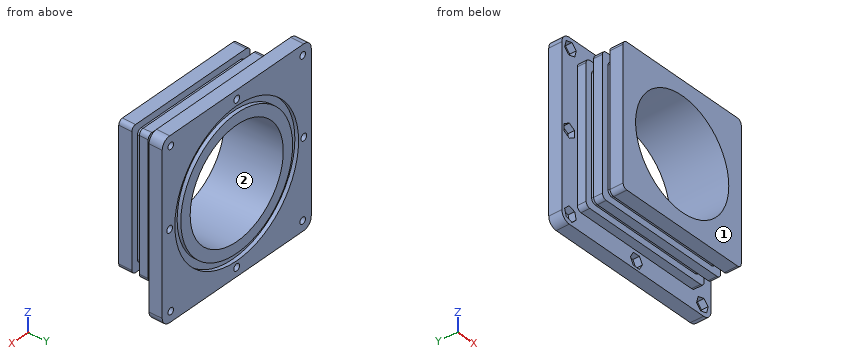
```python
from build123d import *

# Parameters (mm, degrees)
SKETCH_3_W               = 80
SKETCH_3_H               = 80
EXTRUDE_1_DEPTH          = 6
SKETCH_4_W               = 63.4
SKETCH_4_H               = 63.4
EXTRUDE_2_DEPTH          = 4
SKETCH_5_W               = 57.4
SKETCH_5_H               = 57.4
EXTRUDE_3_DEPTH          = 3.45
SKETCH_6_W               = 63.4
SKETCH_6_H               = 63.4
EXTRUDE_4_DEPTH          = 4
SKETCH_7_W               = 57.4
SKETCH_7_H               = 57.4
EXTRUDE_5_DEPTH          = 3.45
SKETCH_8_W               = 63.4
SKETCH_8_H               = 63.4
EXTRUDE_6_DEPTH          = 6
SKETCH_11_R              = 25
CUT_EXTRUDE_3_DEPTH      = 1
CUT_EXTRUDE_3_DEPTH_BACK = 27.9
SKETCH_12_R              = 33.2
SKETCH_12_R_2            = 30
CUT_EXTRUDE_4_DEPTH      = 1.7
SKETCH_13_R              = 1.55
CUT_EXTRUDE_5_DEPTH      = 6
PATTERN_CIRCULAR_1_COUNT = 4
SKETCH_14_R              = 1.5
CUT_EXTRUDE_6_DEPTH      = 6
PATTERN_CIRCULAR_2_COUNT = 4
CUT_EXTRUDE_7_DEPTH      = 3
PATTERN_CIRCULAR_3_COUNT = 4
FILLET_1_R               = 2
FILLET_2_R               = 4


with BuildPart() as part:
    # 草图3 → 凸台-拉伸1 (new body)
    with BuildSketch(Plane(origin=(0, 0, 0), x_dir=(1, 0, 0), z_dir=(0, 1, 0))):
        Rectangle(SKETCH_3_W, SKETCH_3_H)
    extrude(amount=EXTRUDE_1_DEPTH)

    # 草图4 → 凸台-拉伸2 (add)
    with BuildSketch(Plane(origin=(0, 0, 0), x_dir=(-1, 0, 0), z_dir=(0, -1, 0))):
        Rectangle(SKETCH_4_W, SKETCH_4_H)
    extrude(amount=EXTRUDE_2_DEPTH)

    # 草图5 → 凸台-拉伸3 (add)
    with BuildSketch(Plane(origin=(0, -4, 0), x_dir=(-1, 0, 0), z_dir=(0, -1, 0))):
        Rectangle(SKETCH_5_W, SKETCH_5_H)
    extrude(amount=EXTRUDE_3_DEPTH)

    # 草图6 → 凸台-拉伸4 (add)
    with BuildSketch(Plane(origin=(0, -7.45, 0), x_dir=(-1, 0, 0), z_dir=(0, -1, 0))):
        Rectangle(SKETCH_6_W, SKETCH_6_H)
    extrude(amount=EXTRUDE_4_DEPTH)

    # 草图7 → 凸台-拉伸5 (add)
    with BuildSketch(Plane(origin=(0, -11.45, 0), x_dir=(-1, 0, 0), z_dir=(0, -1, 0))):
        Rectangle(SKETCH_7_W, SKETCH_7_H)
    extrude(amount=EXTRUDE_5_DEPTH)

    # 草图8 → 凸台-拉伸6 (add)
    with BuildSketch(Plane(origin=(0, -14.9, 0), x_dir=(-1, 0, 0), z_dir=(0, -1, 0))):
        Rectangle(SKETCH_8_W, SKETCH_8_H)
    extrude(amount=EXTRUDE_6_DEPTH)

    # 草图11 → 切除-拉伸3 (cut, two sides)
    with BuildSketch(Plane(origin=(0, 6, 0), x_dir=(1, 0, 0), z_dir=(0, 1, 0))) as cut_extrude_3_sk:
        Circle(SKETCH_11_R)
    extrude(amount=CUT_EXTRUDE_3_DEPTH, mode=Mode.SUBTRACT)
    extrude(cut_extrude_3_sk.sketch, amount=-CUT_EXTRUDE_3_DEPTH_BACK, mode=Mode.SUBTRACT)

    # 草图12 → 切除-拉伸4 (cut)
    with BuildSketch(Plane(origin=(0, 6, 0), x_dir=(1, 0, 0), z_dir=(0, 1, 0))):
        Circle(SKETCH_12_R)
        Circle(SKETCH_12_R_2, mode=Mode.SUBTRACT)
    extrude(amount=-CUT_EXTRUDE_4_DEPTH, mode=Mode.SUBTRACT)

    # 草图13 → 切除-拉伸5 (cut)
    with BuildSketch(Plane(origin=(0, 6, 0), x_dir=(1, 0, 0), z_dir=(0, 1, 0))):
        with Locations((0, 36)):
            Circle(SKETCH_13_R)
    cut_extrude_5 = extrude(amount=-CUT_EXTRUDE_5_DEPTH, mode=Mode.SUBTRACT)

    # 阵列(圆周)1: 切除-拉伸5 ×4 about axis
    pattern_circular_1_axis = Axis((0, 0, 0), (0, 1, 0))
    for i in range(1, PATTERN_CIRCULAR_1_COUNT):
        add(cut_extrude_5.rotate(pattern_circular_1_axis, i * 360 / PATTERN_CIRCULAR_1_COUNT), mode=Mode.SUBTRACT)

    # 草图14 → 切除-拉伸6 (cut)
    with BuildSketch(Plane(origin=(0, 6, 0), x_dir=(1, 0, 0), z_dir=(0, 1, 0))):
        with Locations((-35.403805922, 35.403805922)):
            Circle(SKETCH_14_R)
    cut_extrude_6 = extrude(amount=-CUT_EXTRUDE_6_DEPTH, mode=Mode.SUBTRACT)

    # 阵列(圆周)2: 切除-拉伸6 ×4 about axis
    pattern_circular_2_axis = Axis((0, 0, 0), (0, 1, 0))
    for i in range(1, PATTERN_CIRCULAR_2_COUNT):
        add(cut_extrude_6.rotate(pattern_circular_2_axis, i * 360 / PATTERN_CIRCULAR_2_COUNT), mode=Mode.SUBTRACT)

    # 草图15 → 切除-拉伸7 (cut)
    with BuildSketch(Plane(origin=(0, 0, 0), x_dir=(-1, 0, 0), z_dir=(0, -1, 0))):
        Polygon((1.615900042, 33.199607101), (3.233161412, 35.999214037), (1.61726137, 38.799606936), (-1.615900042, 38.800392899), (-3.233161412, 36.000785963), (-1.61726137, 33.200393064), align=None)
        Polygon((-37.689996349, 37.689996349), (-38.526800123, 34.567002148), (-36.240609696, 32.280811722), (-33.117615496, 33.117615496), (-32.280811722, 36.240609696), (-34.567002148, 38.526800123), align=None)
    cut_extrude_7 = extrude(amount=-CUT_EXTRUDE_7_DEPTH, mode=Mode.SUBTRACT)

    # 阵列(圆周)3: 切除-拉伸7 ×4 about axis
    pattern_circular_3_axis = Axis((0, 0, 0), (0, 1, 0))
    for i in range(1, PATTERN_CIRCULAR_3_COUNT):
        add(cut_extrude_7.rotate(pattern_circular_3_axis, i * 360 / PATTERN_CIRCULAR_3_COUNT), mode=Mode.SUBTRACT)

    # 圆角1
    fillet_1_edges = [part.edges().sort_by_distance(p)[0] for p in [
        (-31.7, -2, 31.7),
        (-31.7, -2, -31.7),
        (31.7, -2, -31.7),
        (31.7, -2, 31.7),
        (-28.7, -5.725, 28.7),
        (-28.7, -5.725, -28.7),
        (28.7, -5.725, -28.7),
        (28.7, -5.725, 28.7),
        (-31.7, -9.45, 31.7),
        (-31.7, -9.45, -31.7),
        (31.7, -9.45, -31.7),
        (31.7, -9.45, 31.7),
        (-28.7, -13.175, 28.7),
        (-28.7, -13.175, -28.7),
        (28.7, -13.175, -28.7),
        (28.7, -13.175, 28.7),
        (-31.7, -17.9, 31.7),
        (-31.7, -17.9, -31.7),
        (31.7, -17.9, -31.7),
        (31.7, -17.9, 31.7),
    ]]
    fillet(fillet_1_edges, radius=FILLET_1_R)

    # 圆角2
    fillet_2_edges = [part.edges().sort_by_distance(p)[0] for p in [
        (40, 3, 40),
        (-40, 3, 40),
        (-40, 3, -40),
        (40, 3, -40),
    ]]
    fillet(fillet_2_edges, radius=FILLET_2_R)


solid = part.part
```
Read the model definition and answer for the solid it produces. Units are mm, in the model's axes. Face numbers are marked on the shaded views. Round coordinates to 2 decimals unless told otherwise and drop trailing zeros. Loops run counter-clockwise (first coordinate to the right, second up) from the corner with the lowest first, then second, coordinate; pieces in that order, holes last. Notation, with made-up numbers: (-9, 50.5) -> (25, 50.5) arc R22 cw to (25, 87.5) -> close; hole circle Ø7 at (-15, -19.75). An arc over 180 degrees is marked (long way). One line per item, written item: value.
1) Flat-ended cylindrical pins translate along their axes: P1, Ø4, axis at y = -13.5, z = -16, coming from the +X side; P2, Ø12, axis at y = -10.5, z = -5.5, coming from the -X side; P3, Ø1.7, axis at x = 7, y = -14, coming from the -Z side. Find the tip coordinate at first contact, or state that the pin passes through.
Answer list:
P1: stops at x = 31.7
P2: stops at x = -31.7
P3: stops at z = -28.7
2) Consider L1, parallel to Z at x = 0, y = 4.65; L2, parallel to Y at x = 0, z = 29.5. Determine where each line is inside the solid, lowest interval first. Write a range as [from, to].
Answer list:
L1: z = [-40, -37.55], [-34.45, -33.2], [-30, -25], [25, 30], [33.2, 34.45], [37.55, 40]
L2: y = [-20.9, -14.9], [-11.45, -7.45], [-4, 6]
3) The mould has two halves that part along X. Classify the marked faces 1 and 2: pulls with the +X half, pulls with the -X half, needs draft (parallel to the pull), parting line crosses it, or undercut.
Answer list:
face 1: needs draft
face 2: undercut
4) A cutting plane is placed at B-B (z = 0). Give the number of separate pieces and of enclosed holes in the cut face, and give its area (3 significant figures).
Answer list:
separate pieces: 4
enclosed holes: 0
area: 356 mm²
5) A cutting plane is placed at A-A (y = -19). Determine the outline of the cut face in (x, z), and give its area (3 significant figures).
Answer list:
outline: (-31.7, -29.7) arc R2 ccw to (-29.7, -31.7) -> (29.7, -31.7) arc R2 ccw to (31.7, -29.7) -> (31.7, 29.7) arc R2 ccw to (29.7, 31.7) -> (-29.7, 31.7) arc R2 ccw to (-31.7, 29.7) -> close; hole circle Ø50 at (0, 0)
area: 2,050 mm²
